The drawing under review shows one solid part. Ordinate dimensions are in mm from its lowest x, y, z. A direction names the side the tool comes from. Coordinates: 2 decimals unless noted, no trailing zeros. Order: outer loops, then holes, each group sorted by start corner. A loop starts at its lowest first (then second) coordinate and runs counter-clockwise, first axis right, second up.
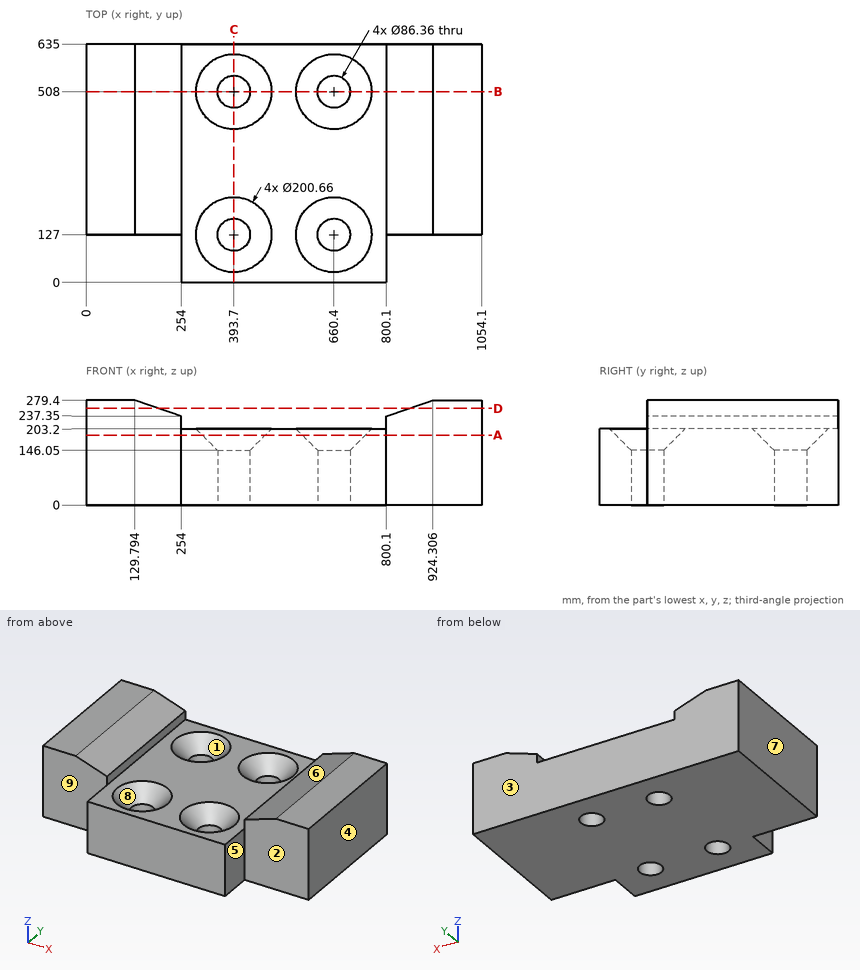
1. Clearance check with flat-ended pins moving along their axes: pin 1 Ø2 at (y, z) = (97, 119) entering from -X; pin 2 Ø8 at (x, y) = (367, 83.5) entering from +Z; pin 3 Ø4 at (x, z) = (888.5, 108) entering from -Y. State where each tip first meets the part, or that it passes through.
Answer below:
pin 1: stops at x = 254
pin 2: stops at z = 157.91
pin 3: stops at y = 127
2. Take a section at B-B, the plane y = 508. Give the boundary of the cut face in (x, z), plus the area to 3 significant figures.
Answer below:
outline: (0, 0) - (350.52, 0) - (350.52, 146.05) - (293.37, 203.2) - (254, 203.2) - (254, 237.35) - (129.79, 279.4) - (0, 279.4) - close; (436.88, 0) - (617.22, 0) - (617.22, 146.05) - (560.07, 203.2) - (494.03, 203.2) - (436.88, 146.05) - close; (703.58, 0) - (1054.1, 0) - (1054.1, 279.4) - (924.31, 279.4) - (800.1, 237.35) - (800.1, 203.2) - (760.73, 203.2) - (703.58, 146.05) - close
area: 206,000 mm2
3. Take a section at D-D, the plane z = 258. Give the boundary of the cut face in (x, y).
Answer below:
outline: (0, 127) - (193, 127) - (193, 635) - (0, 635) - close; (861.1, 127) - (1054.1, 127) - (1054.1, 635) - (861.1, 635) - close
4. Machinability: for the marked faces 5, 6, 7, 8 and 9, which of the approach directions +Z, -Z, +X, -X, +Y, -Y give a long, thin tool a straight path to every point of the face, cutting with its end or side? Answer none if there is none.
Answer below:
face 5: +Z, -Z, +X, -Y
face 6: +Z, +Y, -Y
face 7: +Z, -Z, -X, +Y, -Y
face 8: +Z
face 9: +Z, -Z, -X, -Y
5. Take a section at A-A, the plane z = 187. Give the boundary of the cut face in (x, y).
Answer below:
outline: (0, 127) - (254, 127) - (254, 0) - (800.1, 0) - (800.1, 127) - (1054.1, 127) - (1054.1, 635) - (0, 635) - close; hole circle Ø168.26 at (393.7, 127); hole circle Ø168.26 at (393.7, 508); hole circle Ø168.26 at (660.4, 127); hole circle Ø168.26 at (660.4, 508)
6. Take a section at C-C, the plane x = 393.7. Give the boundary of the cut face in (y, z).
Answer below:
outline: (0, 0) - (83.82, 0) - (83.82, 146.05) - (26.67, 203.2) - (0, 203.2) - close; (170.18, 0) - (464.82, 0) - (464.82, 146.05) - (407.67, 203.2) - (227.33, 203.2) - (170.18, 146.05) - close; (551.18, 0) - (635, 0) - (635, 203.2) - (608.33, 203.2) - (551.18, 146.05) - close
7. The part is to be moulded in two halves that separate along Y. For the marked faces 1, 2, 3 and 4, say which applies: +Y half, -Y half, draft (parallel to the pull), parting line (faces both ways), or undercut.
Answer below:
face 1: undercut
face 2: -Y half
face 3: +Y half
face 4: draft
8. To check wall thickness, follow L1, parallel to X at y = 508, z = 52; L2, parallel to Y at x = 660.4, z = 89.5; L3, parallel to X at y = 359.5, z = 207.5. State the ranges of each line that lie inside material, in increasing order.
Answer below:
L1: x = 0 to 350.52, 436.88 to 617.22, 703.58 to 1054.1
L2: y = 0 to 83.82, 170.18 to 464.82, 551.18 to 635
L3: x = 0 to 254, 800.1 to 1054.1
